```python
from build123d import *

# Parameters (mm, degrees)
F0_W           = 279.4
F0_H           = 25.4
F1_DEPTH       = 3.175
F3_DEPTH       = 25.4
F4_W           = 279.4
F4_H           = 19.05
F5_DEPTH       = 0.3175
F7_D           = 3.6576
F7_CSINK_D     = 7.7978
F7_CSINK_ANGLE = 82


with BuildPart() as f1:
    # F0 (on Top) → F1 (new body, symmetric)
    with BuildSketch(Plane.XY):
        Rectangle(F0_W, F0_H)
    extrude(amount=F1_DEPTH, both=True)

    # F2 (on face) → F3 (cut)
    with BuildSketch(Plane.XZ.offset(12.7)):
        Polygon((139.7, 3.175), (114.3, 3.175), (139.7, -1.5875), align=None)
    extrude(amount=-F3_DEPTH, mode=Mode.SUBTRACT)

    # F4 (on face) → F5 (cut)
    with BuildSketch(Plane(origin=(0, 0, -3.175), x_dir=(1, 0, 0), z_dir=(0, 0, -1))):
        Rectangle(F4_W, F4_H)
    extrude(amount=-F5_DEPTH, mode=Mode.SUBTRACT)

    # F7 (through all)
    with Locations(Plane(origin=(0, 0, -2.8575), x_dir=(1, 0, 0), z_dir=(0, 0, -1))):
        with Locations((-112.7125, 0), (-96.8375, 0)):
            CounterSinkHole(F7_D / 2, F7_CSINK_D / 2, counter_sink_angle=F7_CSINK_ANGLE)


solid = f1.part
```
Build history of the part. All positions in model axes, mm. Round coordinates to 2 decimals unless told otherwise and drop trailing zeros. Loops run counter-clockwise (first coordinate to the right, second up) from the corner with the lowest first, then second, coordinate; pieces in that order, holes last.
Item 1: Drill centre line: line 1 along Z through (x, y) = (54, 6) (1 decimal). Where is it in solid material? Low to high.
Item 2: Two-plate mould, pull along Y, no slides. Class faces 1 (the face through (-2, 0, -2.858)), 2 (the face through (-139.7, 0, 0)), 3 (the face through (-2, 12.7, 0)), 4 (the face through (-95.306, 1.174, -0.592)): released by +Y, released by -Y, zero draft, split by the parting line, or undercut.
Item 3: Pin check, flat tips, straight feed: P1, Ø3.5, axis at x = -112.71, y = 0, coming from the +Z side; P2, Ø1.5, axis at x = 33, y = -7.5, coming from the -Z side. Stop position of each tip, or through.
Item 4: Saw through at B-B (z = 1.25). List the corners of the cut face in (x, y), then the cut area to 3 significant figures.
Worked answers:
1. line 1: z = -2.9 to 3.2
2. face 1: undercut
2. face 2: zero draft
2. face 3: released by +Y
2. face 4: undercut
3. P1: passes through
3. P2: stops at z = -2.86
4. outline: (-139.7, -12.7) - (124.57, -12.7) - (124.57, 12.7) - (-139.7, 12.7) - close; hole circle Ø3.66 at (-112.71, 0); hole circle Ø3.66 at (-96.84, 0)
4. area: 6,690 mm2
